from build123d import *

# Parameters (mm, degrees)
BOSS_EXTRUDE1_DEPTH = 34.925
SKETCH2_R           = 3.175
CUT_EXTRUDE1_DEPTH  = 4.175
SKETCH3_R           = 2.5
CUT_EXTRUDE2_DEPTH  = 39.1


with BuildPart() as part:
    # Sketch1 → Boss-Extrude1 (new body)
    with BuildSketch(Plane.XY):
        Polygon((0, 0), (3.175, 0), (3.175, 34.925), (25.4, 34.925), (25.4, 38.1), (0, 38.1), align=None)
    extrude(amount=BOSS_EXTRUDE1_DEPTH)

    # Sketch2 → Cut-Extrude1 (cut, through all)
    with BuildSketch(Plane(origin=(3.175, 0, 0), x_dir=(0, 0, -1), z_dir=(1, 0, 0))):
        with Locations((-25.4, 12.7)):
            Circle(SKETCH2_R)
        with Locations((-9.525, 12.7)):
            Circle(SKETCH2_R)
    extrude(amount=-CUT_EXTRUDE1_DEPTH, mode=Mode.SUBTRACT)

    # Sketch3 → Cut-Extrude2 (cut, through all)
    with BuildSketch(Plane(origin=(0, 38.1, 0), x_dir=(1, 0, 0), z_dir=(0, 1, 0))):
        with Locations((12.7, -17.4625)):
            Circle(SKETCH3_R)
    extrude(amount=-CUT_EXTRUDE2_DEPTH, mode=Mode.SUBTRACT)


solid = part.part
Geometry: final body of the model. Coordinates: model frame, mm. A direction names the side the tool comes from. Coordinates: 2 decimals unless noted, no trailing zeros. Order: outer loops, then holes, each group sorted by start corner. A loop starts at its lowest first (then second) coordinate and runs counter-clockwise, first axis right, second up.
1) Ray query, probe 1 along Z at (x, y) = (1.25, 13.5) (3 decimals); probe 2 along Y at (x, z) = (1.1, 25.4) (3 decimals); probe 3 along Z at (x, y) = (12.7, 35.7) (1 decimal). Return the intervals inside material, ascending.
Result sheet:
probe 1: z = 0 to 6.452, 12.598 to 22.327, 28.473 to 34.925
probe 2: y = 0 to 9.525, 15.875 to 38.1
probe 3: z = 0 to 15, 20 to 34.9
2) Set-up query: faces 4 (the flat face through (3.175, 17, 17)), 5 (the cylindrical face through (1.61, 10.768, 12.045)). Return all of +Z, -Z, +X, -X, +Y, -Y with unobstructed straight access to the full face (end or side cutting, diameter ignored); none if empty.
Result sheet:
face 4: +Z, -Z, +X, -Y
face 5: +X, -X
3) Draft query along X for faces 1 (the flat face through (0, 19, 17)), 2 (the flat face through (2, 0, 17)), 3 (the cylindrical face through (12.375, 36.535, 14.984)). Return one class per face: released by +X, released by -X, zero draft, split by the parting line, or undercut.
Result sheet:
face 1: released by -X
face 2: zero draft
face 3: undercut
4) Section C-C (z = 18). Return loops of the section in (x, y) (3 decimals).
Result sheet:
outline: (0, 0) - (3.175, 0) - (3.175, 34.925) - (10.258, 34.925) - (10.258, 38.1) - (0, 38.1) - close; (15.142, 34.925) - (25.4, 34.925) - (25.4, 38.1) - (15.142, 38.1) - close
5) Section B-B (y = 12.7). Return loops of the section in (x, z) (3 decimals), then the cut area to 3 significant figures.
Result sheet:
outline: (0, 0) - (3.175, 0) - (3.175, 6.35) - (0, 6.35) - close; (0, 12.7) - (3.175, 12.7) - (3.175, 22.225) - (0, 22.225) - close; (0, 28.575) - (3.175, 28.575) - (3.175, 34.925) - (0, 34.925) - close
area: 70.6 mm2
6) First-contact query: P1, Ø5, axis at y = 23, z = 20.5, coming from the +X side (3 decimals); P2, Ø8, axis at x = 12.7, z = 17.46, coming from the -Y side (3 decimals). Flat tips, straight axial feed; report the tip coordinate or a pass-through.
Result sheet:
P1: stops at x = 3.175
P2: stops at y = 34.925
7) Section D-D (x = 1.75). Return loops of the section in (y, z) (3 decimals), then the cut area to 3 significant figures.
Result sheet:
outline: (0, 0) - (38.1, 0) - (38.1, 34.925) - (0, 34.925) - close; hole circle Ø6.35 at (12.7, 9.525); hole circle Ø6.35 at (12.7, 25.4)
area: 1,270 mm2
8) Section A-A (x = 12.7). Return loops of the section in (y, z) (1 decimal), then the cut area to 3 significant figures.
Result sheet:
outline: (34.9, 0) - (38.1, 0) - (38.1, 15) - (34.9, 15) - close; (34.9, 20) - (38.1, 20) - (38.1, 34.9) - (34.9, 34.9) - close
area: 95.0 mm2
